```python
from build123d import *

# Parameters (mm, degrees)
BOSS_EXTRUDE1_DEPTH = 25.4
CHAMFER1_SIZE       = 19.05
CHAMFER1_SIZE2      = 32.995567884
FILLET1_R           = 6.35


# Read off the part's stored shape, not the designer's step: AdvancedHole1
with BuildPart() as part:
    # Sketch1 → Boss-Extrude1 (new body)
    with BuildSketch(Plane.XY):
        Polygon((0, 0), (0, 19.05), (-38.1, 19.05), (-38.1, 44.45), (63.5, 44.45), (63.5, 19.05), (25.4, 19.05), (25.4, 0), align=None)
    extrude(amount=BOSS_EXTRUDE1_DEPTH)

    # Chamfer1
    chamfer1_edges = [part.edges().sort_by_distance(p)[0] for p in [
        (12.7, 44.45, 25.4),
    ]]
    chamfer1_side = [part.faces().sort_by_distance(p)[0] for p in [
        (12.7, 44.45, 12.7),
    ]]
    chamfer(chamfer1_edges, length=CHAMFER1_SIZE, length2=CHAMFER1_SIZE2, reference=chamfer1_side[0])

    # Fillet1
    # the kernel refuses this fillet: 6.35 mm, written as the material it takes off along each edge
    with BuildSketch(Plane(origin=(-53.975, 44.45, 0), x_dir=(0, -1, 0), z_dir=(1, 0, 0))) as fillet1_piece_1:
        with BuildLine():
            CenterArc((FILLET1_R, -FILLET1_R), FILLET1_R, 90, 90)
            Line((0, -FILLET1_R), (0, 0))
            Line((0, 0), (FILLET1_R, 0))
        make_face()
    extrude(amount=133.35, mode=Mode.SUBTRACT)
    with BuildSketch(Plane(origin=(-47.265435523, 44.45, 6.35), x_dir=(0, -0.8660254037844407, 0.49999999999999656), z_dir=(1, 0, 0))) as fillet1_piece_2:
        with BuildLine():
            CenterArc((FILLET1_R * 0.57735026919, FILLET1_R), FILLET1_R, 210, 60)
            Line((-FILLET1_R * 0.288675134595, FILLET1_R * 0.5), (0, 0))
            Line((0, 0), (FILLET1_R * 0.57735026919, 0))
        make_face()
    extrude(amount=119.930871047, mode=Mode.SUBTRACT)

    # AdvancedHole1 outline → AdvancedHole1 (revolve, cut)
    with BuildSketch(Plane(origin=(12.7, 0, 12.7), x_dir=(1, 0, 0), z_dir=(0, 0, 1))):
        Polygon((8.33374, 0), (8.33374, 12.7), (0, 17.707416175), (0, 0), align=None)
    revolve(axis=Axis((12.7, 0, 12.7), (0, 1, 0)), mode=Mode.SUBTRACT)


solid = part.part
```
The model under review builds one solid part; all positions refer to its coordinate system, in mm. A direction names the side the tool comes from. Give positions to 0.01 mm unless a question says otherwise; leave off trailing zeros. Write each loop counter-clockwise with the first axis right and the second up, starting at its lowest first coordinate (ties: lowest second). Pieces come first, ordered by that corner, then holes. Notation, with made-up numbers: M -35,2 L -5,2 A11 ccw -5,12 Z; hole C 25.5,-8 d6. An arc over 180 degrees is marked long. Write each question's results on one line, items separated by ' | '. Start each with the question number.
1. Insertion check: pin 1 Ø15 at (x, z) = (12.7, 12.7) entering from +Y; pin 2 Ø6.5 at (x, z) = (41, 15) entering from -Y; pin 3 Ø4 at (y, z) = (13.5, 19.5) entering from -X. Each pin has a flat end and moves straight along its axis. Give the tip position at first contact, or say it passes through.
2. We need section B-B (x = -18). Write out the cut boundary in (y, z) (3 decimals), and give its area (3 significant figures).
3. For probe 1 along Z at (x, y) = (12.7, 9.5); probe 2 along X at (y, z) = (15, 15), list the stretches that pass through material, from the lowest coordinate up. Write a range as [from, to].
4. We need section D-D (y = 35). Write out the cut boundary in (x, z).
5. For faces 1 (the cylindrical face through (4.374, 6.439, 12.334)), 2 (the flat face through (45, 19.05, 10)), 3 (the flat face through (0, 9, 13)), list the 3-axis set-ups (+Z, -Z, +X, -X, +Y, -Y) from which the entire face can be reached by the end or side of a thin tool; tool diameter is ignored.
6. We need section A-A (y = 8). Write out the cut boundary in (x, z), and give its area (3 significant figures).
7. Mouldability with a two-part tool opening along X and no side actions: class faces 4 (the conical face through (12.412, 16.908, 13.999)), 5 (the flat face through (63.5, 29, 8)), 6 (the flat face through (13, 24, 0)) as released by +X, released by -X, zero draft, split by the parting line, or undercut.
8. We need section C-C (z = 22.5). Write out the cut boundary in (x, y).
Results found:
1) pin 1: stops at y = 43.93 | pin 2: stops at y = 19.05 | pin 3: stops at x = 0
2) outline: M 19.05,0 L 38.1,0 A6.35 ccw 44.18,4.517 A6.35 ccw 41.275,8.183 L 19.05,21.015 Z | area: 337 mm^2
3) probe 1: z = [0, 4.37], [21.03, 25.4] | probe 2: x = [0, 8.83], [16.57, 25.4]
4) outline: M -38.1,0 L 63.5,0 L 63.5,11.81 L -38.1,11.81 Z
5) face 1: -Y | face 2: +Z, -Z, +X, -Y | face 3: +Z, -Z, -X, -Y
6) outline: M 0,0 L 25.4,0 L 25.4,25.4 L 0,25.4 Z; hole C 12.7,12.7 d16.67 | area: 427 mm^2
7) face 4: undercut | face 5: released by +X | face 6: zero draft
8) outline: M 0,0 L 25.4,0 L 25.4,16.48 L 0,16.48 Z
